Here's how the part is built. I have some questions about the finished solid (model axes, mm). A direction names the side the tool comes from. Give positions to 0.01 mm unless a question says otherwise; leave off trailing zeros. Loops run counter-clockwise (first coordinate to the right, second up) from the corner with the lowest first, then second, coordinate; pieces in that order, holes last. Notation, with made-up numbers: (-11, 16.5) -> (39, 16.5) arc R12 ccw to (39, 26.5) -> close; hole circle Ø2 at (18.25, 44.5). An arc over 180 degrees is marked (long way). Answer in a Markdown table with one row per item. Add a question column.
Item 1: We'd pull the mould along X, two halves only. Please class faces 1 (the face through (125, -32, 54)), 2 (the face through (-115, -29, 49)), 3 (the face through (33, 0, 105)): released by +X, released by -X, zero draft, split by the parting line, or undercut.
Item 2: For P1, Ø8, axis at x = -69.5, z = 102.5, coming from the +Y side; P2, Ø1.5, axis at x = 49.5, z = 23.5, coming from the +Y side; P3, Ø5, axis at x = 6.5, z = 105, coming from the +Y side, each with a flat end and sliding along its axis, tell me the tip position at first contact or that it passes through.
Item 3: Which directions (+Z, -Z, +X, -X, +Y, -Y) give clear straight access to the entire face, cutting with the end or side of a thin tool? Please do faces 4 (the face through (-31, 0, 105)), 5 (the face through (0, -14.434, 105)), 6 (the face through (-70, -25, 105)), 7 (the face through (115, -29, 49)).
Item 4: If we section it at A-A (z = 17): Write out the boundary of the cut face in (x, y), then the cut area to 3 significant figures.
Item 5: If we section it at B-B (y = -19): Write out the boundary of the cut face in (x, z).
Item 6: If I drill on line 1 (X direction, y = -6.5, z = 65.5); line 2 (Y direction, x = 85, z = 57.5); line 3 (Z direction, x = 27, y = -25), over which ranges is the centre line in solid material (lowest first)?
Item 7: If we section it at C-C (x = 75): Write out the boundary of the cut face in (y, z).
Item 8: If we section it at D-D (y = -6): Write out the boundary of the cut face in (x, z), then the cut area to 3 significant figures.
```python
from build123d import *

# Parameters (mm, degrees)
SKETCH1_W               = 250
SKETCH1_H               = 125
SKETCH1_W_2             = 230
SKETCH1_H_2             = 115
BOSS_EXTRUDE1_DEPTH     = 100
SKETCH3_W               = 250
SKETCH3_H               = 125
SKETCH3_W_2             = 230
SKETCH3_H_2             = 115
SKETCH3_R               = 25
SKETCH3_W_3             = 50
SKETCH3_H_3             = 50
BOSS_EXTRUDE4_DEPTH     = 10
CUT_EXTRUDE1_DEPTH      = 178.851764118
CUT_EXTRUDE1_DEPTH_BACK = 178.851764118


with BuildPart() as part:
    # Sketch1 → Boss-Extrude1 (new body)
    with BuildSketch(Plane.XY):
        Rectangle(SKETCH1_W, SKETCH1_H)
        Rectangle(SKETCH1_W_2, SKETCH1_H_2, mode=Mode.SUBTRACT)
    extrude(amount=BOSS_EXTRUDE1_DEPTH)

    # Sketch3 → Boss-Extrude4 (add)
    # profile 1 of 2: a face of its own
    with BuildSketch(Plane.XY.offset(100)):
        Rectangle(SKETCH3_W, SKETCH3_H)
        Rectangle(SKETCH3_W_2, SKETCH3_H_2, mode=Mode.SUBTRACT)
    # profile 2 of 2: a face of its own
    with BuildSketch(Plane.XY.offset(100)):
        Rectangle(SKETCH3_W_2, SKETCH3_H_2)
        with Locations((75, 0)):
            Circle(SKETCH3_R, mode=Mode.SUBTRACT)
        with Locations((-70, 0)):
            Rectangle(SKETCH3_W_3, SKETCH3_H_3, mode=Mode.SUBTRACT)
        Polygon((0, 28.867513459), (25, -14.43375673), (-25, -14.43375673), align=None, mode=Mode.SUBTRACT)
    extrude(amount=BOSS_EXTRUDE4_DEPTH)

    # Sketch4 → Cut-Extrude1 (cut, two sides: drawn at the far end of the back side and taken through both)
    with BuildSketch(Plane.XY.offset(-CUT_EXTRUDE1_DEPTH_BACK)):
        Polygon((-709.844547741, 0), (-138.233831443, 0), (148.761573573, 0), (720.372289871, 0), (720.372289871, 1143.221432596), (-709.844547741, 1143.221432596), align=None)
    extrude(amount=CUT_EXTRUDE1_DEPTH + CUT_EXTRUDE1_DEPTH_BACK, mode=Mode.SUBTRACT)


solid = part.part
```
Recorded:
| question | item | result |
|---|---|---|
| 1 | face 1 | released by +X |
| 1 | face 2 | undercut |
| 1 | face 3 | zero draft |
| 2 | P1 | stops at y = -25 |
| 2 | P2 | stops at y = -57.5 |
| 2 | P3 | stops at y = -14.43 |
| 3 | face 4 | +Z, -Z, +X, -X, +Y |
| 3 | face 5 | +Z, -Z |
| 3 | face 6 | +Z, -Z, +Y |
| 3 | face 7 | -Z, +Y |
| 4 | outline | (-125, -62.5) -> (125, -62.5) -> (125, 0) -> (115, 0) -> (115, -57.5) -> (-115, -57.5) -> (-115, 0) -> (-125, 0) -> close |
| 4 | area | 2,400 mm^2 |
| 5 | outline | (-125, 0) -> (-115, 0) -> (-115, 100) -> (-95, 100) -> (-95, 110) -> (-125, 110) -> close; (-45, 100) -> (58.75, 100) -> (58.75, 110) -> (-45, 110) -> close; (91.25, 100) -> (115, 100) -> (115, 0) -> (125, 0) -> (125, 110) -> (91.25, 110) -> close |
| 6 | line 1 | x = -125 to -115, 115 to 125 |
| 6 | line 2 | y = -62.5 to -57.5 |
| 6 | line 3 | z = 100 to 110 |
| 7 | outline | (-62.5, 0) -> (-57.5, 0) -> (-57.5, 100) -> (-25, 100) -> (-25, 110) -> (-62.5, 110) -> close |
| 8 | outline | (-125, 0) -> (-115, 0) -> (-115, 100) -> (-95, 100) -> (-95, 110) -> (-125, 110) -> close; (-45, 100) -> (-20.13, 100) -> (-20.13, 110) -> (-45, 110) -> close; (20.13, 100) -> (50.73, 100) -> (50.73, 110) -> (20.13, 110) -> close; (99.27, 100) -> (115, 100) -> (115, 0) -> (125, 0) -> (125, 110) -> (99.27, 110) -> close |
| 8 | area | 3,110 mm^2 |
